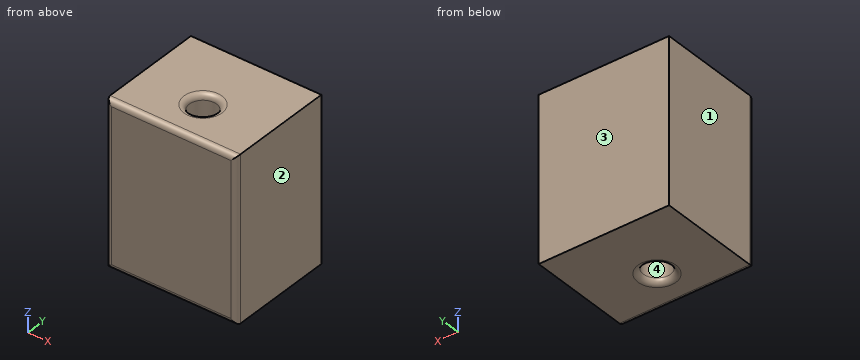
```python
from build123d import *

# Parameters (mm, degrees)
SKETCH1_W               = 24
SKETCH1_H               = 30
BOSS_EXTRUDE1_DEPTH     = 20
CUT_EXTRUDE1_DEPTH      = 44.312815655
CUT_EXTRUDE1_DEPTH_BACK = 44.312815655
SKETCH2_R               = 2.5
FILLET1_R               = 1


with BuildPart() as part:
    # Sketch1 → Boss-Extrude1 (new body)
    with BuildSketch(Plane(origin=(0, 0, 0), x_dir=(1, 0, 0), z_dir=(0, 1, 0))):
        with Locations((12, 15)):
            Rectangle(SKETCH1_W, SKETCH1_H)
    extrude(amount=BOSS_EXTRUDE1_DEPTH)

    # Sketch2 → Cut-Extrude1 (cut, two sides: drawn at the far end of the back side and taken through both)
    with BuildSketch(Plane(origin=(0, 0, -30), x_dir=(-1, 0, 0), z_dir=(0, 0, -1)).offset(-CUT_EXTRUDE1_DEPTH_BACK)):
        with Locations((-12, 7.5)):
            Circle(SKETCH2_R)
    extrude(amount=CUT_EXTRUDE1_DEPTH + CUT_EXTRUDE1_DEPTH_BACK, mode=Mode.SUBTRACT)

    # Fillet1
    fillet1_edges = [part.edges().sort_by_distance(p)[0] for p in [
        (14.5, 7.5, 0),
        (14.5, 7.5, -30),
        (12, 0, -30),
        (24, 0, -15),
        (12, 0, 0),
        (0, 0, -15),
    ]]
    fillet(fillet1_edges, radius=FILLET1_R)


solid = part.part
```
Verification items for the finished model (mm, model axes). Face numbers are marked on the shaded views. Coordinates: 2 decimals unless noted, no trailing zeros. Write each loop counter-clockwise with the first axis right and the second up, starting at its lowest first coordinate (ties: lowest second). Pieces come first, ordered by that corner, then holes. Notation, with made-up numbers: M 88.25,58.25 L 109.25,58.25 A23 cw 109.25,70.25 Z; hole C 28.5,-3 d6. An arc over 180 degrees is marked long. Answer as a JSON object with one key per item and string values. Group by question number.
(1) Cross-section at C-C, the plane x = 12. Record the cut outline in (y, z).
(2) Release check for a two-part mould opening along X. For the marked faces 1, 2, 3 and 4 record: +X half, -X half, draft (parallel to the pull), parting line (faces both ways), or undercut.
(3) Gauge pin test, flat ends, axial feed: pin 1 (8 mm diameter, centred on x = 15.5, y = 9.5, fed in from +Z); pin 2 (4.5 mm diameter, centred on x = 12, y = 7.5, fed in from -Z); pin 3 (1 mm diameter, centred on x = 14, y = 6, fed in from +Z). Record the tip position at first contact, or that the pin passes through.
(4) Cross-section at A-A, the plane z = -19.25. Record the cut outline in (x, y), and give its area (3 significant figures).
(5) Cross-section at B-B, the plane y = 7.5. Record the cut outline in (x, z), and give its area (3 significant figures).
(6) Material ranges on line 1 (Y direction, x = 12, z = -12.25); line 2 (X direction, y = 7.5, z = -21); line 3 (Y direction, x = 9.75, z = -27), recorded low to high.
Reply:
{
 "1": {"outline": "M 0,-29 A1 ccw 1,-30 L 4,-30 A1 ccw 5,-29 L 5,-1 A1 ccw 4,0 L 1,0 A1 ccw 0,-1 Z; M 10,-29 A1 ccw 11,-30 L 20,-30 L 20,0 L 11,0 A1 ccw 10,-1 Z"},
 "2": {"face 1": "-X half", "face 2": "+X half", "face 3": "draft", "face 4": "undercut"},
 "3": {"pin 1": "z = 0", "pin 2": "through", "pin 3": "z = -0.13"},
 "4": {"outline": "M 0,1 A1 ccw 1,0 L 23,0 A1 ccw 24,1 L 24,20 L 0,20 Z; hole C 12,7.5 d5", "area": "460 mm²"},
 "5": {"outline": "M 0,-30 L 8.5,-30 A1 ccw 9.5,-29 L 9.5,-1 A1 ccw 8.5,0 L 0,0 Z; M 14.5,-29 A1 ccw 15.5,-30 L 24,-30 L 24,0 L 15.5,0 A1 ccw 14.5,-1 Z", "area": "569 mm²"},
 "6": {"line 1": "0 to 5, 10 to 20", "line 2": "0 to 9.5, 14.5 to 24", "line 3": "0 to 6.41, 8.59 to 20"}
}
